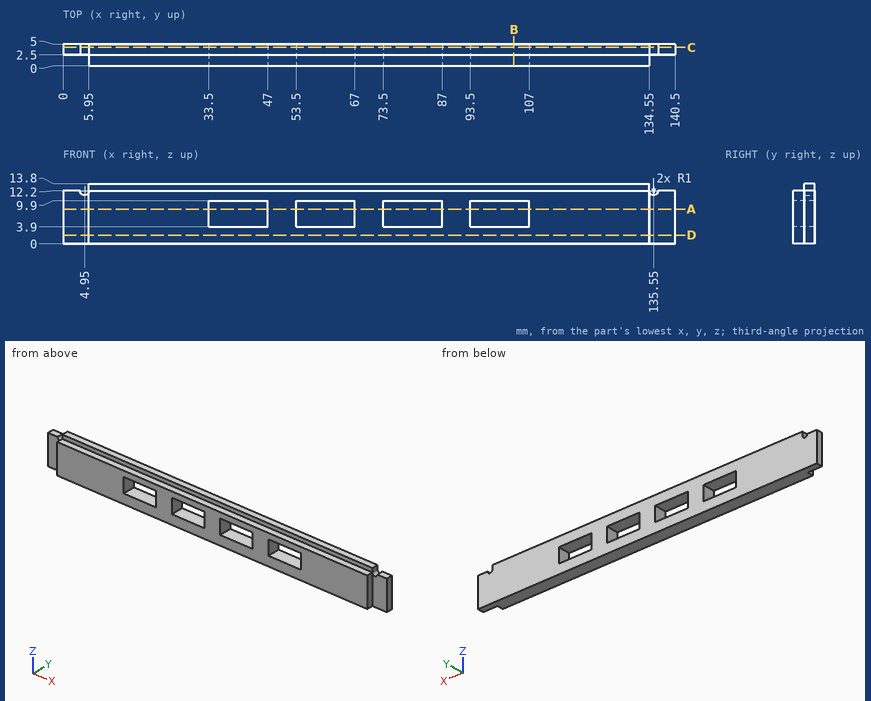
Part print with two shaded views. Sizes in mm from the minimum x, y, z corner. Round coordinates to 2 decimals unless told otherwise and drop trailing zeros. Order: outer loops, then holes, each group sorted by start corner. A loop starts at its lowest first (then second) coordinate and runs counter-clockwise, first axis right, second up. Notation, with made-up numbers: (-28.5, 84.5) -> (-10.5, 84.5) arc R18 cw to (-10.5, 114.5) -> close; hole circle Ø1 at (68, 89.25). An arc over 180 degrees is marked (long way). Write each question's results on one line, items separated by ' | '.
1. Cut at B-B (x = 103.5). Give the cut face in (y, z), plus the area to 3 significant figures.
Findings below:
outline: (0, 0) -> (5, 0) -> (5, 3.9) -> (0, 3.9) -> close; (0, 9.9) -> (5, 9.9) -> (5, 13.8) -> (2.5, 13.8) -> (2.5, 12.2) -> (0, 12.2) -> close | area: 35.0 mm²
2. Cut at C-C (y = 4.25). Give the cut face in (x, z), plus the area to 3 significant figures.
Findings below:
outline: (0, 0) -> (140.5, 0) -> (140.5, 12.2) -> (136.55, 12.2) arc R1 cw to (134.55, 12.2) -> (134.55, 13.8) -> (5.95, 13.8) -> (5.95, 12.2) arc R1 cw to (3.95, 12.2) -> (0, 12.2) -> close; hole (33.5, 3.9) -> (47, 3.9) -> (47, 9.9) -> (33.5, 9.9) -> close; hole (53.5, 3.9) -> (67, 3.9) -> (67, 9.9) -> (53.5, 9.9) -> close; hole (73.5, 3.9) -> (87, 3.9) -> (87, 9.9) -> (73.5, 9.9) -> close; hole (93.5, 3.9) -> (107, 3.9) -> (107, 9.9) -> (93.5, 9.9) -> close | area: 1,590 mm²
3. Cut at D-D (z = 2). Give the cut face in (x, y), plus the area to 3 significant figures.
Findings below:
outline: (0, 2.5) -> (5.95, 2.5) -> (5.95, 0) -> (134.55, 0) -> (134.55, 2.5) -> (140.5, 2.5) -> (140.5, 5) -> (0, 5) -> close | area: 673 mm²
4. Cut at A-A (z = 8). Give the cut face in (x, y), plus the area to 3 significant figures.
Findings below:
outline: (0, 2.5) -> (5.95, 2.5) -> (5.95, 0) -> (33.5, 0) -> (33.5, 5) -> (0, 5) -> close; (47, 0) -> (53.5, 0) -> (53.5, 5) -> (47, 5) -> close; (67, 0) -> (73.5, 0) -> (73.5, 5) -> (67, 5) -> close; (87, 0) -> (93.5, 0) -> (93.5, 5) -> (87, 5) -> close; (107, 0) -> (134.55, 0) -> (134.55, 2.5) -> (140.5, 2.5) -> (140.5, 5) -> (107, 5) -> close | area: 403 mm²
5. Wall check: line 1 along X through (y, z) = (4, 8); line 2 along X through (y, z) = (2.15, 7.5); line 3 along Z through (x, y) = (75, 2.25). Give the ranges that are in metal, low to high. Write a range as [from, to].
Findings below:
line 1: x = [0, 33.5], [47, 53.5], [67, 73.5], [87, 93.5], [107, 140.5] | line 2: x = [5.95, 33.5], [47, 53.5], [67, 73.5], [87, 93.5], [107, 134.55] | line 3: z = [0, 3.9], [9.9, 12.2]
6. Flat gauge pins, fed straight in: P1, Ø3, axis at x = 3, z = 7.5, coming from the -Y side; P2, Ø2, axis at x = 139.5, y = 3, coming from the +Z side; P3, Ø2, axis at y = 1, z = 4.5, coming from the +X side. Where does each tip first touch, or does it go through?
Findings below:
P1: stops at y = 2.5 | P2: stops at z = 12.2 | P3: stops at x = 134.55
